Source: CAD feature listing. Evaluate the final solid. Frame: model axes, mm. A direction names the side the tool comes from. Round coordinates to 2 decimals unless told otherwise and drop trailing zeros. Order: outer loops, then holes, each group sorted by start corner. A loop starts at its lowest first (then second) coordinate and runs counter-clockwise, first axis right, second up. Notation, with made-up numbers: M 39.5,37 L 93.5,37 A16 cw 93.5,58 Z; hole C -39,18 d1. An arc over 180 degrees is marked long. Use CSV: the item, a comma, the result in double quotes. Start each with the question number.
```python
from build123d import *

# Parameters (mm, degrees)
F1_DEPTH = 260.35
F3_DEPTH = 11.90725
F5_DEPTH = 25.4


with BuildPart() as f1:
    # F0 (on Right) → F1 (new body)
    with BuildSketch(Plane.YZ):
        Polygon((11.90625, 0), (0, 0), (0, -483.39375), (-388.9375, -483.39375), (-388.9375, -128.2984649666), (-318.3013850362, -5.953125), (-328.6125, 0), (-400.84375, -125.1081948942), (-400.84375, -495.3), (11.90625, -495.3), align=None)
    extrude(amount=F1_DEPTH)

    # F2 (on Front) → F3 (cut, through all)
    with BuildSketch(Plane.XZ):
        Polygon((260.35, 0), (0, 0), (0, -6.35), align=None)
    extrude(amount=-F3_DEPTH, mode=Mode.SUBTRACT)

    # F4 (on face) → F5 (cut)
    with BuildSketch(Plane(origin=(0, -246.459375, 142.2933865006), x_dir=(1, 0, 0), z_dir=(0, -0.8660254038, 0.5))):
        Polygon((260.35, -164.30625), (0, -164.30625), (0, -170.65625), align=None)
    extrude(amount=-F5_DEPTH, mode=Mode.SUBTRACT)


solid = f1.part
```
(1) Line query: line 1 along Y through (x, z) = (43.5, -260); line 2 along Z through (x, y) = (27, -19); line 3 along Y through (x, z) = (195, -98). Output: solid intervals per line, ascending.
(2) Draft query along Z for faces 3 (the face through (128, -197, -495.3)), 4 (the face through (128.353, -364.223, -61.678)), 5 (the face through (128, -388.938, -308)), 6 (the face through (128, 0, -238)). Return one class per face: pulls with the +Z half, pulls with the -Z half, needs draft (parallel to the pull), parting line crosses it, or undercut.
(3) Contact query for flat-ended pins moving along their axis: P1, Ø10, axis at x = 199, y = -36, coming from the +Z side; P2, Ø5, axis at x = 150.5, z = -118.5, coming from the -Y side. Output: stop coordinate, or through.
(4) Section D-D on y = -294.5. Return loops of the section in (x, z).
(5) Section C-C on x = 232.5. Return loops of the section in (y, z).
(6) Reachability of faces 1 (the face through (128, -192, -483.394)), 2 (the face through (260.35, -195, -485)) from +Z, -Z, +X, -X, +Y, -Y: full face, straight path, thin tool, end or side. Return the list, or none.
(7) Section B-B on y = -354. Return loops of the section in (x, z).
(8) Section A-A on z = -196. Return loops of the section in (x, y).
Results below:
1,line 1,"y = -400.84 to -388.94, 0 to 11.91"
1,line 2,"z = -495.3 to -483.39"
1,line 3,"y = -385.19 to -371.44, 0 to 11.91"
2,face 3,"pulls with the -Z half"
2,face 4,"pulls with the +Z half"
2,face 5,"undercut"
2,face 6,"needs draft"
3,P1,"stops at z = -483.39"
3,P2,"stops at y = -398.47"
4,outline,"M 0,-495.3 L 260.35,-495.3 L 260.35,-483.39 L 0,-483.39 Z"
5,outline,"M -400.84,-495.3 L 11.91,-495.3 L 11.91,-0.68 L 0,-0.68 L 0,-483.39 L -388.94,-483.39 L -388.94,-128.3 L -318.64,-6.54 L -328.95,-0.59 L -400.84,-125.11 Z"
6,face 1,"+X, -X"
6,face 2,"+Z, -Z, +X, +Y, -Y"
7,outline,"M 0,-495.3 L 260.35,-495.3 L 260.35,-483.39 L 0,-483.39 Z; M 0,-67.78 L 260.35,-67.78 L 260.35,-43.97 L 0,-43.97 Z"
8,outline,"M 0,-400.84 L 260.35,-400.84 L 260.35,-388.94 L 0,-388.94 Z; M 0,0 L 260.35,0 L 260.35,11.91 L 0,11.91 Z"
